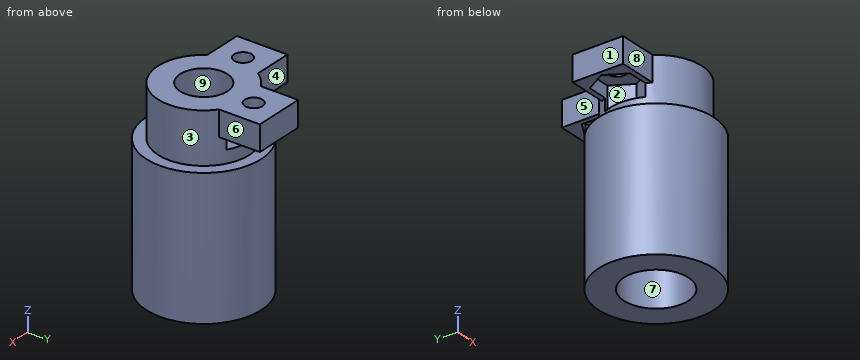
Autodesk Inventor part; units mm, degrees
ref_plane "YZ Plane" through (0, 0, 0) normal (1, 0, 0) x (0, 1, 0)
ref_plane "XZ Plane" through (0, 0, 0) normal (0, 1, 0) x (-1, 0, 0)
ref_plane "XY Plane" through (0, 0, 0) normal (0, 0, 1) x (1, 0, 0)
sketch "Sketch1" plane through (0, 0, 0) normal (0, 0, 1) x (1, 0, 0)
  circle A0 centre (0, 0) radius 6.346
  circle A1 centre (0, 0) radius 11.346
  circle A2 centre (0, 0) radius 4.675
  circle A3 centre (0, 0) radius 9.0554
  dimension "d0" = 12.692
  dimension "d1" = 5
  dimension "d2" = 9.35
  dimension "d7" = 2.7094
extrude "Extrusion1" add sketch "Sketch1" against normal blind 27.225 contours A1 | A3
extrude "Extrusion3" add sketch "Sketch1" along normal blind 10 contours A0 | A3
sketch "Sketch2" plane through (0, 0, 10) normal (0, 0, 1) x (1, 0, 0)
  line L0 (0.5, 10.2508) -> (5.5, 10.2508)
  line L1 (0.5, 10.2508) -> (-4.5, 10.2508)
  line L2 (0.5, 10.2508) -> (0.5, 15.2508)
  line L3 (-10.263, -0.0122) -> (-10.263, 4.9878)
  line L4 (-10.263, -0.0122) -> (-15.263, -0.0122)
  line L5 (-10.263, -0.0122) -> (-10.263, -5.0122)
  line L6 (-10.263, 4.9878) -> (-7.5579, 4.9878)
  circle A0 centre (0, 0) radius 9.0554
  line L7 (-10.263, 4.9878) -> (-15.263, 4.9878)
  line L8 (-15.263, 4.9878) -> (-15.263, -0.0122)
  line L9 (-10.263, -5.0122) -> (-7.5417, -5.0122)
  line L10 (-10.263, -5.0122) -> (-15.263, -5.0122)
  line L11 (-15.263, -5.0122) -> (-15.263, -0.0122)
  line L12 (0.5, 15.2508) -> (5.5, 15.2508)
  line L13 (5.5, 15.2508) -> (5.5, 10.2508)
  line L14 (5.5, 10.2508) -> (5.5, 7.1937)
  line L15 (0.5, 15.2508) -> (-4.5, 15.2508)
  line L16 (-4.5, 15.2508) -> (-4.5, 10.2508)
  line L17 (-4.5, 7.8581) -> (-4.5, 10.2508)
  dimension "d10" = 10.263
  dimension "d11" = 10.263
  dimension "d12" = 5
  dimension "d13" = 5
  dimension "d14" = 5
  dimension "d15" = 5
  dimension "d16" = 5
  dimension "d17" = 5
  dimension "d18" = 15.763
  dimension "d19" = 10.263
extrude "Extrusion4" add sketch "Sketch2" against normal blind 5 contours L2 L12 L13 L0 | L0 L14 A0 L17 L1 | L1 L16 L15 L2 | A0 L9 L5 L3 L6 | L3 L4 L8 L7 | L10 L11 L4 L5
sketch "Sketch4" plane through (0, 0, 5) normal (0, 0, -1) x (-1, 0, 0)
  line L0 (-5.5, 15.2508) -> (4.5, 15.2508)
  line L1 (-0.5, 15.2508) -> (-0.5, 9.7508)
  line L2 (3.5, 7.4414) -> (-0.5, 5.132)
  line L3 (-0.5, 5.132) -> (-4.5, 7.4414)
  line L4 (-4.5, 7.4414) -> (-4.5, 12.0602)
  line L5 (-4.5, 12.0602) -> (-0.5, 14.3696)
  line L6 (-0.5, 14.3696) -> (3.5, 12.0602)
  line L7 (3.5, 12.0602) -> (3.5, 7.4414)
  point P0 (0, 0)
  point P1 (3.5, 9.7508)
  dimension "d22" = 5.5
  dimension "d23" = 8
extrude "Extrusion5" cut sketch "Sketch4" along normal mid plane 5
sketch "Sketch5" plane through (0, 0, 5) normal (0, 0, -1) x (-1, 0, 0)
  line L0 (15.263, 4.9878) -> (15.263, -5.0122)
  line L1 (15.263, -0.0122) -> (9.763, -0.0122)
  line L2 (7.4536, -4.0122) -> (5.1442, -0.0122)
  line L3 (5.1442, -0.0122) -> (7.4536, 3.9878)
  line L4 (7.4536, 3.9878) -> (12.0724, 3.9878)
  line L5 (12.0724, 3.9878) -> (14.3818, -0.0122)
  line L6 (14.3818, -0.0122) -> (12.0724, -4.0122)
  line L7 (12.0724, -4.0122) -> (7.4536, -4.0122)
  line L8 (3.5, 12.0602) -> (3.5, 7.4414)
  point P0 (0, 0)
  dimension "d26" = 5.5
extrude "Extrusion6" cut sketch "Sketch5" along normal mid plane 5
hole "Hole1" at (0.5, 10.2508, 10) at (-10.263, -0.0122, 10) direction (0, 0, -1) diameter 3.5 depth 6.25 tip angle 118
properties part number "springHolder_final"
Check sheet for the modelled part. Datum: model origin and axes. Units: mm. Face numbers are marked on the shaded views. A direction names the side the tool comes from. Round coordinates to 2 decimals unless told otherwise and drop trailing zeros. Order: outer loops, then holes, each group sorted by start corner. A loop starts at its lowest first (then second) coordinate and runs counter-clockwise, first axis right, second up. Notation, with made-up numbers: (-37, 10.5) -> (4, 10.5) arc R11 cw to (4, 17.5) -> close; hole circle Ø11 at (0, 12.5). An arc over 180 degrees is marked (long way). One line per item, written item: value. Start each with the question number.
Q1. Thickness scan on line 1 (Y direction, x = 0.5, z = 8.55); line 2 (Z direction, x = -9.25, y = -2.25) (3 decimals); line 3 (Y direction, x = 0, z = 6.25) (3 decimals). Record the ranges inside material, lowest first.
Q2. Gauge pin test, flat ends, axial feed: pin 1 Ø1.4 at (x, z) = (-10.5, 5.5) entering from -Y; pin 2 Ø4 at (x, z) = (-6.5, 0.5) entering from +Y; pin 3 Ø4 at (x, z) = (-6, -7) entering from -Y; pin 4 Ø8 at (y, z) = (3, -20) entering from +X. Record the tip position at first contact, or that the pin passes through.
Q3. Mould release check, pull along X, two halves, no side actions. Record for the marked faces 1, 2, 3 and 4: pulls with the +X half, pulls with the -X half, needs draft (parallel to the pull), parting line crosses it, or undercut.
Q4. Cross-section at C-C (z = -3.5). Record the boundary of the cut face in (x, y), and give its area (3 significant figures).
Q5. Set-up check for the marked faces 5, 6, 7, 8 and 9: record each of +Z, -Z, +X, -X, +Y, -Y from which the full face is reachable in a straight line by a thin tool's end or side.
Q6. Cross-section at A-A (y = 1). Record the boundary of the cut face in (x, z) (3 decimals).
Q7. Cross-section at D-D (y = -2.5). Record the boundary of the cut face in (x, z) (3 decimals), and give its area (3 significant figures).
Q8. Cross-section at B-B (x = 2.75). Record the boundary of the cut face in (y, z) (3 decimals), and give its area (3 significant figures).
Completed:
1. line 1: y = -9.04 to -4.65, 4.65 to 8.5, 12 to 15.25
1. line 2: z = -27.225 to 0, 7.5 to 10
1. line 3: y = -9.055 to -4.675, 4.675 to 5.421, 14.081 to 15.251
2. pin 1: stops at y = -5.01
2. pin 2: stops at y = 10.39
2. pin 3: stops at y = -10.62
2. pin 4: stops at x = 11.35
3. face 1: pulls with the -X half
3. face 2: undercut
3. face 3: parting line crosses it
3. face 4: needs draft
4. outline: circle Ø22.69 at (0, 0); hole circle Ø12.69 at (0, 0)
4. area: 278 mm²
5. face 5: +Z, -X, +Y
5. face 6: +Z, +X, +Y
5. face 7: -Z
5. face 8: +Z, -X, -Y
5. face 9: +Z, -Z
6. outline: (-15.263, 5) -> (-13.797, 5) -> (-13.797, 7.5) -> (-11.691, 7.5) -> (-11.691, 10) -> (-15.263, 10) -> close; (-11.302, -27.225) -> (-6.267, -27.225) -> (-6.267, 0) -> (-4.567, 0) -> (-4.567, 10) -> (-8.835, 10) -> (-8.835, 7.5) -> (-5.729, 7.5) -> (-5.729, 2.5) -> (-9, 2.5) -> (-9, 0) -> (-11.302, 0) -> close; (4.567, 0) -> (6.267, 0) -> (6.267, -27.225) -> (11.302, -27.225) -> (11.302, 0) -> (9, 0) -> (9, 10) -> (4.567, 10) -> close
7. outline: (-15.263, 5) -> (-12.945, 5) -> (-12.945, 7.5) -> (-6.581, 7.5) -> (-6.581, 2.5) -> (-8.703, 2.5) -> (-8.703, 0) -> (-11.067, 0) -> (-11.067, -27.225) -> (-5.833, -27.225) -> (-5.833, 0) -> (-3.95, 0) -> (-3.95, 10) -> (-15.263, 10) -> close; (3.95, 0) -> (5.833, 0) -> (5.833, -27.225) -> (11.067, -27.225) -> (11.067, 0) -> (8.703, 0) -> (8.703, 10) -> (3.95, 10) -> close
7. area: 392 mm²
8. outline: (-11.008, -27.225) -> (-5.719, -27.225) -> (-5.719, 0) -> (-3.781, 0) -> (-3.781, 10) -> (-8.628, 10) -> (-8.628, 0) -> (-11.008, 0) -> close; (3.781, 0) -> (5.719, 0) -> (5.719, -27.225) -> (11.008, -27.225) -> (11.008, 0) -> (8.628, 0) -> (8.628, 2.5) -> (6.431, 2.5) -> (6.431, 7.5) -> (13.071, 7.5) -> (13.071, 5) -> (15.251, 5) -> (15.251, 10) -> (3.781, 10) -> close
8. area: 396 mm²
